from build123d import *

# Parameters (mm, degrees)
SKETCH_1_R          = 2
SKETCH_1_R_2        = 1.5
EXTRUDE_1_DEPTH     = 2.5
SKETCH_2_R          = 2
CUT_EXTRUDE_1_DEPTH = 2.5
SKETCH_3_R          = 1.5
EXTRUDE_2_DEPTH     = 2


with BuildPart() as part:
    # 草图1 → 凸台-拉伸1 (new, symmetric)
    with BuildSketch(Plane.XY):
        Polygon((0, 0), (60.033704039, -20.01123468), (100.056173399, 0), (100.056173399, 20.015752082), (60.056173399, 40.015752082), (0, 19.997027615), align=None)
        with Locations((20, 5)):
            Circle(SKETCH_1_R, mode=Mode.SUBTRACT)
        with Locations((20, 15)):
            Circle(SKETCH_1_R, mode=Mode.SUBTRACT)
        with Locations((49, 5)):
            Circle(SKETCH_1_R, mode=Mode.SUBTRACT)
        with Locations((49, 15)):
            Circle(SKETCH_1_R, mode=Mode.SUBTRACT)
        with Locations((90, 17)):
            Circle(SKETCH_1_R_2, mode=Mode.SUBTRACT)
        with Locations((90, 3)):
            Circle(SKETCH_1_R_2, mode=Mode.SUBTRACT)
    extrude(amount=EXTRUDE_1_DEPTH, both=True)

    # 草图2 → 切除-拉伸1 (cut, symmetric)
    with BuildSketch(Plane.XY):
        with Locations((80, 10)):
            Circle(SKETCH_2_R)
        with Locations((4, 5)):
            Circle(SKETCH_2_R)
        with Locations((4, 15)):
            Circle(SKETCH_2_R)
    extrude(amount=CUT_EXTRUDE_1_DEPTH, both=True, mode=Mode.SUBTRACT)

    # 草图3 → 凸台-拉伸2 (add)
    with BuildSketch(Plane.XY.offset(2.5)):
        with BuildLine():
            Line((92.5, 17), (92.5, 3))
            ThreePointArc((92.5, 3), (90, 0.5), (87.5, 3))
            Line((87.5, 3), (87.5, 17))
            ThreePointArc((87.5, 17), (90, 19.5), (92.5, 17))
        make_face()
        with Locations((90, 17)):
            Circle(SKETCH_3_R, mode=Mode.SUBTRACT)
        with Locations((90, 3)):
            Circle(SKETCH_3_R, mode=Mode.SUBTRACT)
    extrude(amount=EXTRUDE_2_DEPTH)


solid = part.part
The listing builds one solid part. Answer for the finished solid, in the listing's coordinates (mm). A direction names the side the tool comes from. Coordinates: 2 decimals unless noted, no trailing zeros. Write each loop counter-clockwise with the first axis right and the second up, starting at its lowest first coordinate (ties: lowest second). Pieces come first, ordered by that corner, then holes. Notation, with made-up numbers: (72, -28) - (112, -28) arc R14 cw to (112, -4) - close; hole circle Ø5 at (29.5, 61.5). An arc over 180 degrees is marked (long way). Answer as CSV lines item,"result".
1. Find section C-C (x = 90). Give the vertices of the cut face in (y, z).
Computed values:
outline,"(-5.03, -2.5) - (1.5, -2.5) - (1.5, 4.5) - (0.5, 4.5) - (0.5, 2.5) - (-5.03, 2.5) - close; (4.5, -2.5) - (15.5, -2.5) - (15.5, 4.5) - (4.5, 4.5) - close; (18.5, -2.5) - (25.04, -2.5) - (25.04, 2.5) - (19.5, 2.5) - (19.5, 4.5) - (18.5, 4.5) - close"
2. Determine the mould class of faces 1 (the cylindrical face through (47, 5, 0)), 2 (the cylindrical face through (18, 5, 0)), 3 (the flat face through (100.056, 10, 0)), 4 (the flat face through (30, -10, 0)) for opening direction X: +X half, -X half, draft (parallel to the pull), parting line (faces both ways), or undercut.
Computed values:
face 1,"undercut"
face 2,"undercut"
face 3,"+X half"
face 4,"-X half"
3. Find section D-D (y = 26). Give the vertices of the cut face in (x, z).
Computed values:
outline,"(18.01, -2.5) - (88.09, -2.5) - (88.09, 2.5) - (18.01, 2.5) - close"
4. Find section A-A (z = -0.5). Give the number of separate pieces and of enclosed holes in the cut face, plus the area to 3 significant figures.
Computed values:
separate pieces,"1"
enclosed holes,"9"
area,"3,900 mm²"
5. Find section B-B (x = 4). Give the vertices of the cut face in (y, z).
Computed values:
outline,"(-1.33, -2.5) - (3, -2.5) - (3, 2.5) - (-1.33, 2.5) - close; (7, -2.5) - (13, -2.5) - (13, 2.5) - (7, 2.5) - close; (17, -2.5) - (21.33, -2.5) - (21.33, 2.5) - (17, 2.5) - close"
6. Straight lines are drawn through the part: line 1 (Y direction, x = 90, z = 0); line 2 (Y direction, x = 4, z = -1.1); line 3 (Z direction, x = 42.5, y = 9.5). For each, find the intervals that lie inside material, in ascending order. Write a range as [from, to].
Computed values:
line 1,"y = [-5.03, 1.5], [4.5, 15.5], [18.5, 25.04]"
line 2,"y = [-1.33, 3], [7, 13], [17, 21.33]"
line 3,"z = [-2.5, 2.5]"
7. A tool of negligible diameter and unlimited length cuts with its end or side. For faces 5 (the cylindrical face through (49, 17, 0)), 6 (the cylindrical face through (90.1, 0.5, 3.5)), 7 (the cylindrical face through (89.9, 19.5, 3.5)), from which of +Z, -Z, +X, -X, +Y, -Y can it reach the whole face along a straight path? Write none if from no direction.
Computed values:
face 5,"+Z, -Z"
face 6,"+Z, -Y"
face 7,"+Z, +Y"
8. Given P1, Ø2.5, axis at x = 49, y = 15, coming from the -Z side; P2, Ø3.5, axis at x = 90, y = 17, coming from the +Z side; P3, Ø5, axis at x = 20, y = 15, coming from the +Z side; P4, Ø3, axis at x = 42, z = 1.5, coming from the +Y side, each flat-ended and moving along its own axis, determine where each tip first touches the part or whether it passes through.
Computed values:
P1,"passes through"
P2,"stops at z = 4.5"
P3,"stops at z = 2.5"
P4,"stops at y = 34.5"
